from build123d import *

# Parameters (mm, degrees)
F0_R     = 22.5
F1_DEPTH = 120
F3_DEPTH = 70
F4_R     = 20
F5_DEPTH = 35
F8_D     = 5


with BuildPart() as f1:
    # F0 (on Top) → F1 (new body)
    with BuildSketch(Plane.XY):
        Circle(F0_R)
    extrude(amount=F1_DEPTH)

    # F2 (on face) → F3 (cut)
    with BuildSketch(Plane.XY.offset(120)):
        with BuildLine():
            ThreePointArc((12.5, 18.708287), (0, 22.5), (-12.5, 18.708287))
            Line((-12.5, 18.708287), (-12.5, -18.708287))
            ThreePointArc((-12.5, -18.708287), (0, -22.5), (12.5, -18.708287))
            Line((12.5, -18.708287), (12.5, 18.708287))
        make_face()
    extrude(amount=-F3_DEPTH, mode=Mode.SUBTRACT)

    # F4 (on face) → F5 (cut)
    with BuildSketch(Plane.XY):
        Circle(F4_R)
    extrude(amount=F5_DEPTH, mode=Mode.SUBTRACT)

    # F8 (through all)
    with Locations(Plane.YZ.offset(22.5)):
        with Locations((0, 100)):
            Hole(F8_D / 2)


solid = f1.part
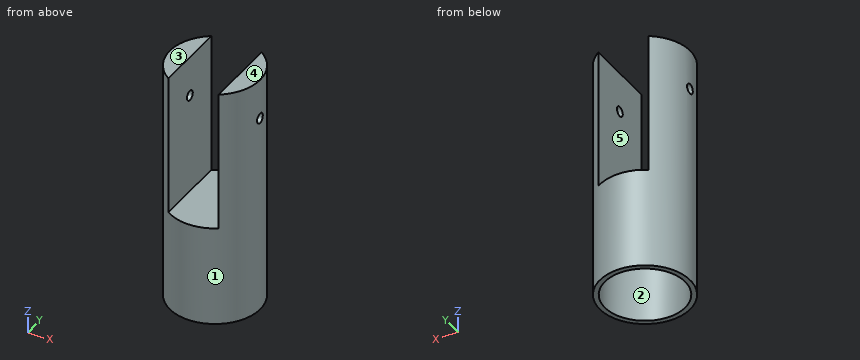
For this review, take the finished solid that the model builds, in its own axes (mm). Face numbers are marked on the shaded views. A direction names the side the tool comes from. Coordinates: 2 decimals unless noted, no trailing zeros. Order: outer loops, then holes, each group sorted by start corner. A loop starts at its lowest first (then second) coordinate and runs counter-clockwise, first axis right, second up. Notation, with made-up numbers: (44.5, 71) -> (99.5, 71) arc R10 cw to (99.5, 79) -> close; hole circle Ø5 at (2, -32). An arc over 180 degrees is marked (long way). Return JSON: item names as keys, results as strings.
1. We need section A-A on y = 0. Write out the cut boundary in (x, z).
Answer block:
{"outline": "(-22.5, 0) -> (-20, 0) -> (-20, 35) -> (20, 35) -> (20, 0) -> (22.5, 0) -> (22.5, 97.5) -> (12.5, 97.5) -> (12.5, 50) -> (-12.5, 50) -> (-12.5, 97.5) -> (-22.5, 97.5) -> close; (-22.5, 102.5) -> (-12.5, 102.5) -> (-12.5, 120) -> (-22.5, 120) -> close; (12.5, 102.5) -> (22.5, 102.5) -> (22.5, 120) -> (12.5, 120) -> close"}
2. We need section B-B on x = 0. Write out the cut boundary in (y, z), and give its area (3 significant figures).
Answer block:
{"outline": "(-22.5, 0) -> (-20, 0) -> (-20, 35) -> (20, 35) -> (20, 0) -> (22.5, 0) -> (22.5, 50) -> (-22.5, 50) -> close", "area": "850 mm²"}
3. We need section D-D on z = 15. Write out the cut boundary in (x, y).
Answer block:
{"outline": "circle Ø45 at (0, 0); hole circle Ø40 at (0, 0)"}
4. The part is to be moulded in two halves that separate along X. For the marked faces 1, 2 and 3, say which applies: +X half, -X half, draft (parallel to the pull), parting line (faces both ways), or undercut.
Answer block:
{"face 1": "parting line", "face 2": "undercut", "face 3": "draft"}
5. Machinability: for the marked faces 4 and 5, which of the approach directions +Z, -Z, +X, -X, +Y, -Y give a long, thin tool a straight path to every point of the face, cutting with its end or side? Answer none if there is none.
Answer block:
{"face 4": "+Z, +X, -X, +Y, -Y", "face 5": "+Z, +Y, -Y"}
6. For line 1 (Y direction, x = 0, z = 19); line 2 (Y direction, x = 18, z = 100); line 3 (Z direction, x = -2, y = -15), list the stretches that pass through material, from the lowest coordinate up. Write a range as from..to.
Answer block:
{"line 1": "-22.5..-20, 20..22.5", "line 2": "-13.5..-2.5, 2.5..13.5", "line 3": "35..50"}
7. We need section C-C on z = 91. Write out the cut boundary in (x, y), and give its area (3 significant figures).
Answer block:
{"outline": "(-12.5, -18.71) -> (-12.5, 18.71) arc R22.5 ccw to start; (12.5, -18.71) arc R22.5 ccw to (12.5, 18.71) -> close", "area": "526 mm²"}
8. For pin 1 Ø8 at (y, z) = (17.5, 29.5) entering from -X; pin 2 Ø1.5 at (x, y) = (11.5, -14.5) entering from -Z; pin 3 Ø6 at (y, z) = (-5, 58.5) entering from -X; pin 4 Ø4 at (y, z) = (0, 100) entering from +X, all flat-tipped, find the tip position at first contact; note any pin that passes through.
Answer block:
{"pin 1": "x = -18", "pin 2": "z = 35", "pin 3": "x = -22.41", "pin 4": "through"}
